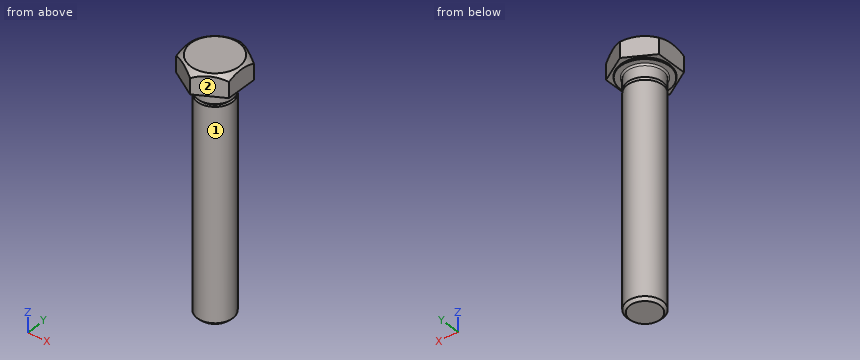
from build123d import *

# Parameters (mm, degrees)
DODANIE_WYCI_GNI_CIE1_DEPTH = 8.2
ZAOKR_GLENIE1_R             = 0.1
SFAZOWANIE1_SIZE            = 1.0825
ZAOKR_GLENIE3_R             = 0.6


with BuildPart() as part:
    # Szkic1 → Dodanie-wyciągnięcie1 (new body)
    with BuildSketch(Plane(origin=(0, 0, 0.6), x_dir=(-1, 0, 0), z_dir=(0, 0, -1))):
        Polygon((4.896e-06, 12.124341521), (-10.499990209, 6.062166521), (-10.499990209, -6.062183479), (-9.791e-06, -12.12435), (10.499990209, -6.062183479), (10.499990209, 6.062166521), align=None)
    extrude(amount=-DODANIE_WYCI_GNI_CIE1_DEPTH)

    # Szkic2 → Obrót1 (revolve)
    with BuildSketch(Plane(origin=(0, 0, 0), x_dir=(1, 0, 0), z_dir=(0, 1, 0))):
        Polygon((7, 90), (0, 90), (0, -0.6), (9.685, -0.6), (9.685, 0), (7, 0), (7, 4.9175), (5.9175, 6), (7, 6), align=None)
    revolve(axis=Axis((0, 0, -90), (0, 0, 1)))

    # Zaokrąglenie1
    zaokr_glenie1_edges = [part.edges().sort_by_distance(p)[0] for p in [
        (-9.685, 0, 0),
    ]]
    fillet(zaokr_glenie1_edges, radius=ZAOKR_GLENIE1_R)

    # Sfazowanie1
    sfazowanie1_edges = [part.edges().sort_by_distance(p)[0] for p in [
        (-7, 0, -90),
    ]]
    chamfer(sfazowanie1_edges, length=SFAZOWANIE1_SIZE)

    # Zaokrąglenie3
    zaokr_glenie3_edges = [part.edges().sort_by_distance(p)[0] for p in [
        (-7, 0, 0),
    ]]
    fillet(zaokr_glenie3_edges, radius=ZAOKR_GLENIE3_R)

    # Szkic3 → Wycięcie-obrót1 (revolve, cut)
    with BuildSketch(Plane(origin=(0, 0, 0), x_dir=(1, 0, 0), z_dir=(0, 1, 0))):
        with BuildLine():
            ThreePointArc((-17, 4.7), (-12.313708499, -6.613708499), (-1, -11.3))
            Line((-1, -11.3), (-17, -11.3))
            Line((-17, -11.3), (-17, 4.7))
        make_face()
        with BuildLine():
            ThreePointArc((-1, -11.3), (-12.313708499, -6.613708499), (-17, 4.7))
            Line((-17, 4.7), (-17, -11.3))
            Line((-17, -11.3), (-1, -11.3))
        make_face()
    revolve(axis=Axis((0, 0, -88.9175), (0, 0, 1)), mode=Mode.SUBTRACT)


solid = part.part
Source: CAD feature listing. Evaluate the final solid. Frame: model axes, mm. Face numbers are marked on the shaded views. A direction names the side the tool comes from. Coordinates: 2 decimals unless noted, no trailing zeros. Loops run counter-clockwise (first coordinate to the right, second up) from the corner with the lowest first, then second, coordinate; pieces in that order, holes last. Notation, with made-up numbers: (-17.5, 68) - (20.5, 68) arc R9 cw to (20.5, 82) - close; hole circle Ø8 at (70, 74). An arc over 180 degrees is marked (long way). One line per item, written item: value. Start each with the question number.
1. Ray query, L1, parallel to Z at x = -4.25, y = 7.5; L2, parallel to Y at x = -0.25, z = -54; L3, parallel to X at y = 3.75, z = -47. Return the intervals inside material, ascending.
2. Set-up query: the marked faces 1 and 2. Return all of +Z, -Z, +X, -X, +Y, -Y with unobstructed straight access to the full face (end or side cutting, diameter ignored); none if empty.
3. Section A-A (z = -32). Return the cut outline in (x, y), and give its area (3 significant figures).
4. Contact query for flat-ended pins moving along their axis: P1, Ø1, axis at x = -7, y = -2.5, coming from the -Z side; P2, Ø6, axis at y = -7, z = -32, coming from the +X side; P3, Ø12, axis at y = 6.5, z = -43.5, coming from the +X side. Output: stop coordinate, or through.
Verdict:
1. L1: z = 0 to 8.8
1. L2: y = -7 to 7
1. L3: x = -5.91 to 5.91
2. face 1: -Z
2. face 2: +Z, -Z, +X, -Y
3. outline: circle Ø14 at (0, 0)
3. area: 154 mm2
4. P1: stops at z = -88.98
4. P2: stops at x = 5.74
4. P3: stops at x = 6.98
